from build123d import *

# Parameters (mm, degrees)
SKETCH1_W          = 48.5
SKETCH1_H          = 44.9
SKETCH2_R          = 4.125
CUT_EXTRUDE1_DEPTH = 26.4
FILLET1_R          = 4.7


with BuildPart() as part:
    # Sketch1 → Revolve1 (revolve)
    with BuildSketch(Plane(origin=(0, 0, 0), x_dir=(1, 0, 0), z_dir=(0, 1, 0))):
        with Locations((24.25, 22.45)):
            Rectangle(SKETCH1_W, SKETCH1_H)
    revolve(axis=Axis((0, 0, 0), (0, 0, -1)))

    # Sketch2 → Cut-Extrude1 (cut)
    with BuildSketch(Plane(origin=(0, 0, -44.9), x_dir=(-1, 0, 0), z_dir=(0, 0, -1))):
        Circle(SKETCH2_R)
    extrude(amount=-CUT_EXTRUDE1_DEPTH, mode=Mode.SUBTRACT)

    # Fillet1
    fillet1_edges = [part.edges().sort_by_distance(p)[0] for p in [
        (-48.5, 0, -44.9),
        (-48.5, 0, 0),
    ]]
    fillet(fillet1_edges, radius=FILLET1_R)


solid = part.part
Build history of the part. All positions in model axes, mm. A direction names the side the tool comes from. Coordinates: 2 decimals unless noted, no trailing zeros. Order: outer loops, then holes, each group sorted by start corner. A loop starts at its lowest first (then second) coordinate and runs counter-clockwise, first axis right, second up. Notation, with made-up numbers: (-20, 70) - (-3, 70) arc R11 ccw to (-3, 77) - close; hole circle Ø4 at (-16, -34). An arc over 180 degrees is marked (long way). Write item = value, one per line. Start each with the question number.
1) Saw through at C-C on z = -21.5. Write the cut outline in (x, y) (3 decimals).
2) Flat gauge pins, fed straight in: pin 1 Ø1.5 at (x, z) = (23, -19.5) entering from -Y; pin 2 Ø6 at (y, z) = (35.5, -23) entering from -X; pin 3 Ø8 at (x, y) = (33.5, 20) entering from +Z; pin 4 Ø5 at (x, z) = (29, -8.5) entering from -Y. Where does each tip first touch, or does it go through?
3) Two-plate mould, pull along Y, no slides. Class faces 1 (the face through (22.38, 43.028, -22.698)), 2 (the face through (1, -1, 0)), 3 (the face through (-3.8, -1.6, -31.9)): pulls with the +Y half, pulls with the -Y half, needs draft (parallel to the pull), parting line crosses it, or undercut.
4) 3-axis set-ups, long thin cutter, end or side, ignore diameter. For faces 4 (the face through (0, 0, -18.5)), 5 (the face through (-9, -1, -44.9)): which of +Z, -Z, +X, -X, +Y, -Y reach the whole face in a straight line?
5) Saw through at D-D on z = -10.5. Write the cut outline in (x, y), then the cut area to 3 significant figures.
6) Saw through at A-A on y = 0. Write the cut outline in (x, z) (3 decimals).
7) Wall check: line 1 along Y through (x, z) = (0, -28) (3 decimals); line 2 along Y through (x, z) = (-27, -39); line 3 along Y through (x, z) = (-28, -8). Give the ranges that are in metal, low to high. Write a range as from..to.
From the geometry:
q1.outline = circle Ø97 at (0, 0); hole circle Ø8.25 at (0, 0)
q2.pin_1 = -43.1
q2.pin_2 = -36
q2.pin_3 = 0
q2.pin_4 = -40.62
q3.face_1 = parting line crosses it
q3.face_2 = needs draft
q3.face_3 = undercut
q4.face_4 = -Z
q4.face_5 = -Z, +X, -X, +Y, -Y
q5.outline = circle Ø97 at (0, 0)
q5.area = 7,390 mm^2
q6.outline = (-48.5, -40.2) arc R4.7 ccw to (-43.8, -44.9) - (-4.125, -44.9) - (-4.125, -18.5) - (4.125, -18.5) - (4.125, -44.9) - (43.8, -44.9) arc R4.7 ccw to (48.5, -40.2) - (48.5, -4.7) arc R4.7 ccw to (43.8, 0) - (-43.8, 0) arc R4.7 ccw to (-48.5, -4.7) - close
q7.line_1 = -48.5..-4.125, 4.125..48.5
q7.line_2 = -40.29..40.29
q7.line_3 = -39.6..39.6
